Source: three-view drawing plus pictorial views. Frame: mm from the lowest corner of the part. Give positions to 0.01 mm unless a question says otherwise; leave off trailing zeros. Loops run counter-clockwise (first coordinate to the right, second up) from the corner with the lowest first, then second, coordinate; pieces in that order, holes last. Notation, with made-up numbers: (61.5, 23.25) -> (106.5, 23.25) arc R17 cw to (106.5, 33.25) -> close; hole circle Ø10 at (15, 13.5). An arc over 180 degrees is marked (long way). Put each result on its own line as item: value.
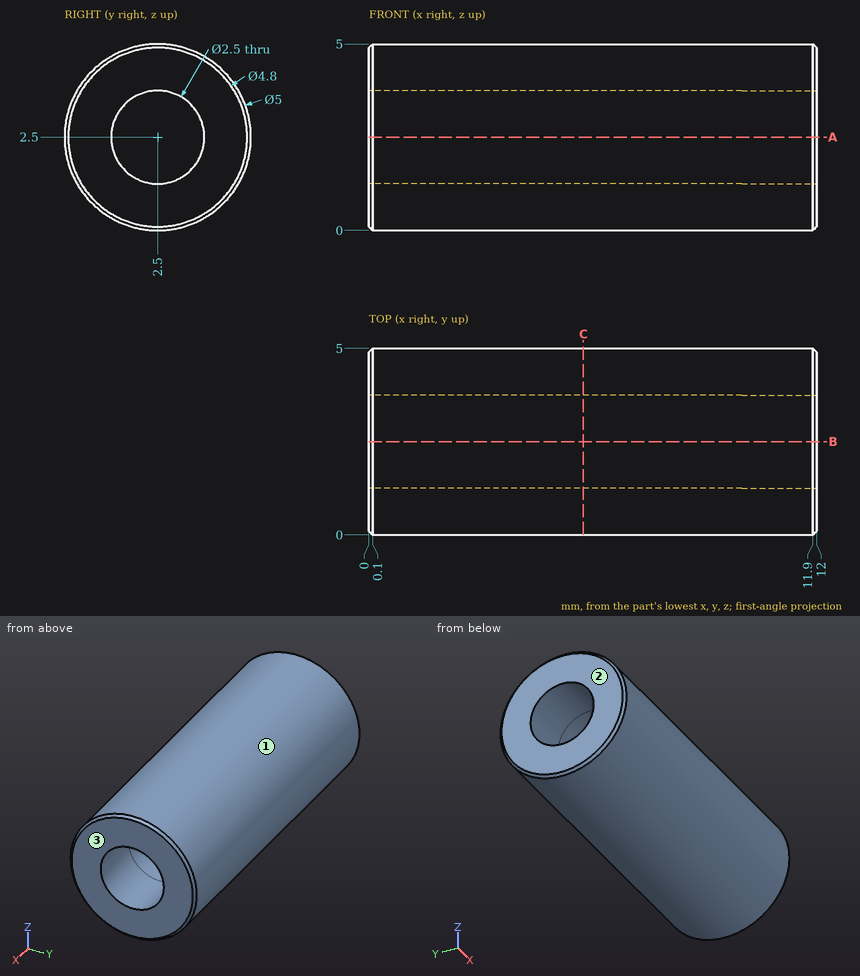
(1) Line query: probe 1 along Z at (x, y) = (4.5, 2.5); probe 2 along Z at (x, y) = (9.5, 1.5); probe 3 along Z at (x, y) = (1, 4). Output: solid intervals per line, ascending. Write a range as from..to.
Calculated:
probe 1: z = 0..1.25, 3.75..5
probe 2: z = 0.21..1.75, 3.25..4.79
probe 3: z = 0.5..4.5
(2) Draft query along X for the marked faces 1, 2 and 3. Return one class per face: released by +X, released by -X, zero draft, split by the parting line, or undercut.
Calculated:
face 1: zero draft
face 2: released by -X
face 3: released by +X
(3) Section A-A on z = 2.5. Return loops of the section in (x, y).
Calculated:
outline: (0, 0.1) -> (0.1, 0) -> (11.9, 0) -> (12, 0.1) -> (12, 1.25) -> (0, 1.25) -> close; (0, 3.75) -> (12, 3.75) -> (12, 4.9) -> (11.9, 5) -> (0.1, 5) -> (0, 4.9) -> close
(4) Section C-C on x = 5.75. Return loops of the section in (y, z).
Calculated:
outline: circle Ø5 at (2.5, 2.5); hole circle Ø2.5 at (2.5, 2.5)
(5) First-contact query: P1, Ø3, axis at y = 2.5, z = 2.5, coming from the -X side; P2, Ø1, axis at x = 10, z = 3.5, coming from the +Y side; P3, Ø1.5, axis at x = 2, z = 4.5, coming from the +Y side. Flat tips, straight axial feed; report the tip coordinate or a pass-through.
Calculated:
P1: stops at x = 0
P2: stops at y = 4.95
P3: stops at y = 4.67
